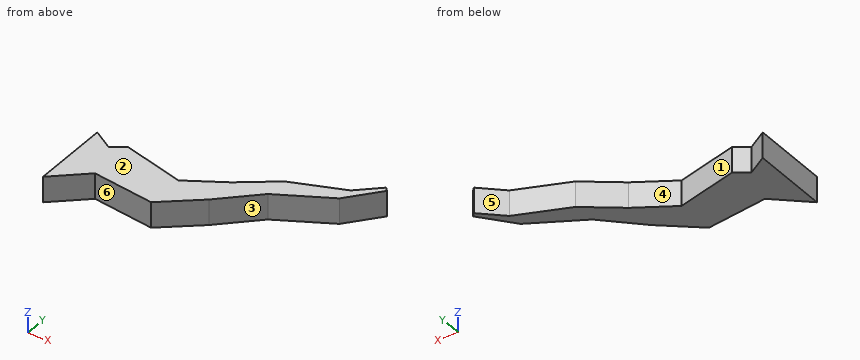
```python
from build123d import *

# Parameters (mm, degrees)
AUFSATZ_LINEAR_AUSTRAGEN1_DEPTH = 3


with BuildPart() as part:
    # Model → Aufsatz-Linear austragen1 (new body)
    with BuildSketch(Plane.XY):
        Polygon((27.757201613, 17.823879819), (25.269410576, 15.48201919), (19.285403887, 13.008865595), (15.246732761, 9.937624528), (10.945087096, 7.248053638), (3.864948468, 8.895369168), (2.346139264, 7.811699181), (0.1, 9.139176818), (0.1, 0.224829603), (3.809633928, 3.57004156), (10.895315766, 2.844989185), (15.122386477, 6.402986505), (19.174325502, 10.407995412), (25.148627395, 13.799695492), (28.124071775, 17.440721322), align=None)
    extrude(amount=AUFSATZ_LINEAR_AUSTRAGEN1_DEPTH)


solid = part.part
```
Input: part model. Units: mm. Frame: model coordinates. Face numbers are marked on the shaded views. A direction names the side the tool comes from. Round coordinates to 2 decimals unless told otherwise and drop trailing zeros. Write each loop counter-clockwise with the first axis right and the second up, starting at its lowest first coordinate (ties: lowest second). Pieces come first, ordered by that corner, then holes. Notation, with made-up numbers: (-16.75, -2) - (22.25, -2) arc R30 ccw to (22.25, 32) - close; hole circle Ø6 at (77.25, 33). An arc over 180 degrees is marked (long way). Write item = value, one per line.
(1) Material intervals for probe 1 along X at (y, z) = (5.5, 0.25); probe 2 along Y at (x, z) = (17.5, 2.75); probe 3 along X at (y, z) = (11.75, 1.55), sorted ascending.
Geometry check:
probe_1 = 0.1 to 14.05
probe_2 = 8.75 to 11.65
probe_3 = 17.63 to 21.54
(2) Pull-direction query (X, two-part tool) for the marked faces 1, 2 and 3; classes: +X half, -X half, draft (parallel to the pull), parting line (faces both ways), or undercut.
Geometry check:
face_1 = undercut
face_2 = draft
face_3 = +X half
(3) Section query A-A on z = 1.25. Output: boundary loops of the cut face in (x, y), then the cut area to 3 significant figures.
Geometry check:
outline = (0.1, 0.22) - (3.81, 3.57) - (10.9, 2.84) - (15.12, 6.4) - (19.17, 10.41) - (25.15, 13.8) - (28.12, 17.44) - (27.76, 17.82) - (25.27, 15.48) - (19.29, 13.01) - (15.25, 9.94) - (10.95, 7.25) - (3.86, 8.9) - (2.35, 7.81) - (0.1, 9.14) - close
area = 103 mm^2
(4) Section query C-C on y = 13.5. Output: boundary loops of the cut face in (x, z).
Geometry check:
outline = (20.47, 0) - (24.62, 0) - (24.62, 3) - (20.47, 3) - close
(5) Access query for the marked faces 4, 5 and 6. Directions: +Z, -Z, +X, -X, +Y, -Y. A direction counts if a zero-diameter tool reaches every point of the face in a straight line with its end or side. Return the directions, or none.
Geometry check:
face_4 = +Z, -Z, +Y
face_5 = +Z, -Z, -X, +Y
face_6 = +Z, -Z, -Y
(6) Section query B-B on x = 10. Output: boundary loops of the cut face in (y, z), then the cut area to 3 significant figures.
Geometry check:
outline = (2.94, 0) - (7.47, 0) - (7.47, 3) - (2.94, 3) - close
area = 13.6 mm^2
(7) Contact query for flat-ended pins moving along their axis: pin 1 Ø4 at (x, y) = (6.5, 6.5) entering from -Z; pin 2 Ø1.5 at (x, z) = (5.5, 0.5) entering from -Y; pin 3 Ø1 at (y, z) = (7, 2) entering from +X; pin 4 Ø1.5 at (x, z) = (4.5, 0.5) entering from +Y. Output: stop coordinate, or through.
Geometry check:
pin_1 = 0
pin_2 = 3.32
pin_3 = 16.23
pin_4 = 8.9
